Check sheet for the modelled part. Datum: model origin and axes. Units: mm. Give positions to 0.01 mm unless a question says otherwise; leave off trailing zeros. Order: outer loops, then holes, each group sorted by start corner. A loop starts at its lowest first (then second) coordinate and runs counter-clockwise, first axis right, second up.
```python
from build123d import *

# Parameters (mm, degrees)
SKETCH_1_R      = 1.75
EXTRUDE_1_DEPTH = 4


with BuildPart() as part:
    # ｽｹｯﾁ1 → ﾎﾞｽ - 押し出し1 (new body)
    with BuildSketch(Plane.XY):
        Polygon((0, 0), (40, 0), (80, 0), (80, 140), (0, 140), align=None)
        with Locations((5, 135)):
            Circle(SKETCH_1_R, mode=Mode.SUBTRACT)
        with Locations((5, 5)):
            Circle(SKETCH_1_R, mode=Mode.SUBTRACT)
        with BuildLine():
            ThreePointArc((40, 41.6), (46.6, 35), (40, 28.4))
            ThreePointArc((40, 28.4), (33.4, 35), (40, 41.6))
        make_face(mode=Mode.SUBTRACT)
        with Locations((75, 5)):
            Circle(SKETCH_1_R, mode=Mode.SUBTRACT)
        with Locations((5, 75)):
            Circle(SKETCH_1_R, mode=Mode.SUBTRACT)
        with Locations((32.25, 90.576606241)):
            Circle(SKETCH_1_R, mode=Mode.SUBTRACT)
        with Locations((32.25, 117.423393759)):
            Circle(SKETCH_1_R, mode=Mode.SUBTRACT)
        with Locations((75, 75)):
            Circle(SKETCH_1_R, mode=Mode.SUBTRACT)
        with BuildLine():
            ThreePointArc((34.440448115, 113.629426332), (45.326056233, 114.075), (39.497374059, 104.870573668))
            ThreePointArc((39.497374059, 104.870573668), (34.673943767, 107.925), (34.440448115, 113.629426332))
        make_face(mode=Mode.SUBTRACT)
        with Locations((55.5, 104)):
            Circle(SKETCH_1_R, mode=Mode.SUBTRACT)
        with Locations((75, 135)):
            Circle(SKETCH_1_R, mode=Mode.SUBTRACT)
    extrude(amount=EXTRUDE_1_DEPTH)


solid = part.part
```
(1) Cross-section at C-C on y = 111. Enter the section's corners in (x, z).
Response values:
outline: (0, 0) - (33.85, 0) - (33.85, 4) - (0, 4) - close; (46.15, 0) - (80, 0) - (80, 4) - (46.15, 4) - close
(2) Material ranges on L1, parallel to Y at x = 75, z = 3.2; L2, parallel to X at y = 111, z = 1.4; L3, parallel to Y at x = 36, z = 3.5, recorded low to high.
Response values:
L1: y = 0 to 3.25, 6.75 to 73.25, 76.75 to 133.25, 136.75 to 140
L2: x = 0 to 33.85, 46.15 to 80
L3: y = 0 to 29.75, 40.25 to 106.33, 115.67 to 140
(3) Cross-section at D-D on x = 55.5. Enter the section's corners in (y, z), then the cut area to 3 significant figures.
Response values:
outline: (0, 0) - (102.25, 0) - (102.25, 4) - (0, 4) - close; (105.75, 0) - (140, 0) - (140, 4) - (105.75, 4) - close
area: 546 mm2
(4) Cross-section at B-B on y = 75. Enter the section's corners in (x, z), then the cut area to 3 significant figures.
Response values:
outline: (0, 0) - (3.25, 0) - (3.25, 4) - (0, 4) - close; (6.75, 0) - (73.25, 0) - (73.25, 4) - (6.75, 4) - close; (76.75, 0) - (80, 0) - (80, 4) - (76.75, 4) - close
area: 292 mm2
(5) Gauge pin test, flat ends, axial feed: pin 1 Ø4 at (x, y) = (32.25, 90.58) entering from -Z; pin 2 Ø3 at (x, y) = (5, 135) entering from -Z. Record the tip position at first contact, or that the pin passes through.
Response values:
pin 1: stops at z = 0
pin 2: passes through
(6) Release check for a two-part mould opening along X. For faces 1 (the face through (39, 71, 0)), 2 (the face through (32.02, 92.31, 1.97)), 3 (the face through (0, 71, 2)) record: released by +X, released by -X, zero draft, split by the parting line, or undercut.
Response values:
face 1: zero draft
face 2: undercut
face 3: released by -X
(7) Cross-section at A-A on x = 5. Enter the section's corners in (y, z), then the cut area to 3 significant figures.
Response values:
outline: (0, 0) - (3.25, 0) - (3.25, 4) - (0, 4) - close; (6.75, 0) - (73.25, 0) - (73.25, 4) - (6.75, 4) - close; (76.75, 0) - (133.25, 0) - (133.25, 4) - (76.75, 4) - close; (136.75, 0) - (140, 0) - (140, 4) - (136.75, 4) - close
area: 518 mm2
